Build history of the part. All positions in model axes, mm. A direction names the side the tool comes from. Give positions to 0.01 mm unless a question says otherwise; leave off trailing zeros. Order: outer loops, then holes, each group sorted by start corner. A loop starts at its lowest first (then second) coordinate and runs counter-clockwise, first axis right, second up. Notation, with made-up numbers: M -2,80 L 21,80 A12 ccw 21,95 Z; hole C 41,-11.75 d8. An arc over 180 degrees is marked long. Use CSV: the item, a comma, the result in double quotes. Start each with the question number.
Item 1: Two-plate mould, pull along X, no slides. Class faces 6 (the flat face through (-88.067, -1.4, 552.416)), 7 (the flat face through (-219.242, -1.4, 717.713)), 8 (the flat face through (265, -1, 470.773)): pulls with the +X half, pulls with the -X half, needs draft (parallel to the pull), parting line crosses it, or undercut.
Item 2: Band-saw the part on C-C on z = -112.5. Write the cut outline in (x, y), plus the area to 3 significant figures.
Item 3: Which spindle directions (+Z, -Z, +X, -X, +Y, -Y) get a long thin tool onto all of the face, cutting with end or side? Do faces 1 (the flat face through (195.467, -1.4, -79.269)), 2 (the cylindrical face through (-55.5, -110.35, 1151.27)), 3 (the flat face through (-35.611, -1, 988)), 4 (the flat face through (-222, -1, -439.137)), 5 (the flat face through (-154.21, -1.4, 636.43)). Say none if no direction does.
Item 4: Band-saw the part on B-B on y = -37. Write the cut outline in (x, z).
Item 5: Pin check, flat tips, straight feed: P1, Ø5, axis at y = 18, z = 907, coming from the +X side; P2, Ø18, axis at y = -36.5, z = 1001, coming from the +X side; P3, Ø4, axis at x = 87.5, y = -50.5, coming from the +Z side. Stop position of each tip, or through.
Item 6: Band-saw the part on A-A on x = -199. Write the cut outline in (y, z), plus the area to 3 significant figures.
Item 7: Band-saw the part on D-D on z = 1002. Write the cut outline in (x, y), plus the area to 3 significant figures.
Item 8: Wall check: line 1 along X through (y, z) = (-59, 708); line 2 along X through (y, z) = (7, 631.5); line 3 along Y through (x, z) = (-134.5, 875.5). Give the ranges that are in metal, low to high.
from build123d import *

# Parameters (mm, degrees)
F1_DEPTH = 100
F2_R     = 21.5886417048
F2_R_2   = 24.6150282736
F3_DEPTH = 21


with BuildPart() as f1:
    # F0 (on Front) → F1 (new body, symmetric)
    with BuildSketch(Plane.XZ):
        with BuildLine():
            ThreePointArc((35.6107763946, 1017.418384552), (98.3474680479, 1128.9674460156), (0, 1210.8628739806))
            ThreePointArc((0, 1210.8628739806), (-98.3474680479, 1128.9674460156), (-35.6107763946, 1017.418384552))
            Line((-35.6107763946, 1017.418384552), (-35.6107763946, 957.8346954225))
            Line((-35.6107763946, 957.8346954225), (-124.767777348, 957.8346954225))
            Line((-124.767777348, 957.8346954225), (-316.3984388356, 470.7734332918))
            Line((-316.3984388356, 470.7734332918), (-248.2028006078, 470.7734332918))
            Line((-248.2028006078, 470.7734332918), (-57.5520955026, 806.7892193794))
            Line((-57.5520955026, 806.7892193794), (-119.449198246, 290.8188700676))
            Line((-119.449198246, 290.8188700676), (-269.3851142813, -439.1371260194))
            Line((-269.3851142813, -439.1371260194), (-173.8435637442, -439.1371260194))
            Line((-173.8435637442, -439.1371260194), (0, 262.8727257252))
            Line((0, 262.8727257252), (173.8435637442, -439.1371260194))
            Line((173.8435637442, -439.1371260194), (269.3851142813, -439.1371260194))
            Line((269.3851142813, -439.1371260194), (119.449198246, 290.8188700676))
            Line((119.449198246, 290.8188700676), (75.1282572746, 803.9661645889))
            Line((75.1282572746, 803.9661645889), (214.4739990169, 470.7734332918))
            Line((214.4739990169, 470.7734332918), (316.3984388356, 470.7734332918))
            Line((316.3984388356, 470.7734332918), (124.767777348, 957.8346954225))
            Line((124.767777348, 957.8346954225), (35.6107763946, 957.8346954225))
            Line((35.6107763946, 957.8346954225), (35.6107763946, 1017.418384552))
        make_face()
    extrude(amount=F1_DEPTH, both=True)

    # F2 (on face) → F3 (join)
    with BuildSketch(Plane.XZ.offset(100)):
        with Locations((-52.6945628226, 1129.8661231995)):
            Circle(F2_R)
        with Locations((35.6107763946, 1156.6877365112)):
            Circle(F2_R_2)
        with BuildLine():
            add(Edge.make_bspline(
                [(-56.1959594488, 1072.7338790894), (-55.924177507, 1059.9617369508), (-16.9304138442, 1031.8550429672), (52.9069858404, 1052.444888033), (68.8536482627, 1100.9438511252), (46.6390210232, 1083.2507084319), (20.7228541214, 1060.5728618004), (-39.3811416258, 1046.8222391451), (-42.433383012, 1098.137824899), (-56.3583007079, 1080.3629571017), (-56.1959594488, 1072.7338790894)],
                knots=[0, 0, 0, 0, 0.1448792193, 0.3216273429, 0.4396148241, 0.51965969, 0.6525806211, 0.7994169759, 0.9134604944, 1, 1, 1, 1], degree=3))
        make_face()
    extrude(amount=F3_DEPTH)


solid = f1.part
Model answer:
1,face 6,"undercut"
1,face 7,"pulls with the -X half"
1,face 8,"needs draft"
2,outline,"M -202.29,-100 L -92.96,-100 L -92.96,100 L -202.29,100 Z; M 92.96,-100 L 202.29,-100 L 202.29,100 L 92.96,100 Z"
2,area,"43,700 mm^2"
3,face 1,"+X, +Y, -Y"
3,face 2,"-Y"
3,face 3,"-X, +Y, -Y"
3,face 4,"-Z, +X, -X, +Y, -Y"
3,face 5,"+Y, -Y"
4,outline,"M -316.4,470.77 L -248.2,470.77 L -57.55,806.79 L -119.45,290.82 L -269.39,-439.14 L -173.84,-439.14 L 0,262.87 L 173.84,-439.14 L 269.39,-439.14 L 119.45,290.82 L 75.13,803.97 L 214.47,470.77 L 316.4,470.77 L 124.77,957.83 L 35.61,957.83 L 35.61,1017.42 A100 ccw long -35.61,1017.42 L -35.61,957.83 L -124.77,957.83 Z"
5,P1,"stops at x = 145.75"
5,P2,"stops at x = 35.61"
5,P3,"stops at z = 1162.73"
6,outline,"M -100,-439.14 L 100,-439.14 L 100,-96.47 L -100,-96.47 Z; M -100,557.49 L 100,557.49 L 100,769.16 L -100,769.16 Z"
6,area,"111,000 mm^2"
7,outline,"M -35.61,-100 L 35.61,-100 L 35.61,100 L -35.61,100 Z"
7,area,"14,200 mm^2"
8,line 1,"x = -223.06 to -113.6, -69.4 to 83.42, 115.26 to 223.06"
8,line 2,"x = -253.16 to -157.01, -78.58 to 90.02, 147.26 to 253.16"
8,line 3,"y = -100 to 100"
